Can you work these out from the model? Positions are in its coordinate system, mm. A direction names the side the tool comes from. Give positions to 0.01 mm unless a question says otherwise; leave off trailing zeros. Write each loop counter-clockwise with the first axis right and the second up, starting at its lowest first coordinate (ties: lowest second). Pieces come first, ordered by that corner, then holes. Notation, with made-up numbers: (9.5, 65.5) - (58.5, 65.5) arc R16 cw to (58.5, 88.5) - close; hole circle Ø8 at (-4, 33.5). An arc over 180 degrees is marked (long way). Use a Markdown table: item, result. Add a question column.
```python
from build123d import *

# Parameters (mm, degrees)
BOSS_EXTRUDE1_DEPTH = 128.5
SKETCH7_W           = 30
SKETCH7_H           = 20
BOSS_EXTRUDE4_DEPTH = 3
CUT_EXTRUDE1_REACH  = 145.152
SKETCH9_R           = 2.5
SKETCH10_W          = 20
SKETCH10_H          = 30
BOSS_EXTRUDE5_DEPTH = 3
CUT_EXTRUDE2_REACH  = 145.753
SKETCH11_R          = 2.5


with BuildPart() as part:
    # Sketch4 → Boss-Extrude1 (new, symmetric)
    with BuildSketch(Plane.XY):
        with BuildLine():
            Line((0, 0), (27, 0))
            Line((27, 0), (27, -3))
            Line((27, -3), (26.800082477, -3))
            ThreePointArc((26.800082477, -3), (-19.135504983, -19.08508544), (-3, 26.83281573))
            Line((-3, 26.83281573), (-3, 27))
            Line((-3, 27), (0, 27))
            Line((0, 27), (0, 0))
        make_face()
    extrude(amount=BOSS_EXTRUDE1_DEPTH, both=True)

    # Sketch7 → Boss-Extrude4 (add)
    with BuildSketch(Plane(origin=(0, 27, 0), x_dir=(1, 0, 0), z_dir=(0, 1, 0))):
        with Locations((12, -43.5)):
            Rectangle(SKETCH7_W, SKETCH7_H)
        with Locations((12, 43.5)):
            Rectangle(SKETCH7_W, SKETCH7_H)
    extrude(amount=BOSS_EXTRUDE4_DEPTH)

    # Sketch9 → Cut-Extrude1 (cut, up to next)
    with BuildSketch(Plane(origin=(0, 30, 0), x_dir=(1, 0, 0), z_dir=(0, 1, 0)), mode=Mode.PRIVATE) as cut_extrude1_sk1:
        with Locations(Location((17, -43.5, 0), (0, 0, 270))):
            Circle(SKETCH9_R)
    cut_extrude1_tool1 = extrude(cut_extrude1_sk1.sketch, amount=-CUT_EXTRUDE1_REACH, mode=Mode.PRIVATE) & part.part
    # Sketch9 → Cut-Extrude1 (cut, up to next)
    with BuildSketch(Plane(origin=(0, 30, 0), x_dir=(1, 0, 0), z_dir=(0, 1, 0)), mode=Mode.PRIVATE) as cut_extrude1_sk2:
        with Locations(Location((17, 43.5, 0), (0, 0, 270))):
            Circle(SKETCH9_R)
    cut_extrude1_tool2 = extrude(cut_extrude1_sk2.sketch, amount=-CUT_EXTRUDE1_REACH, mode=Mode.PRIVATE) & part.part
    add(cut_extrude1_tool1.solids().sort_by_distance((17, 30, 43.5))[0], mode=Mode.SUBTRACT)
    add(cut_extrude1_tool2.solids().sort_by_distance((17, 30, -43.5))[0], mode=Mode.SUBTRACT)

    # Sketch10 → Boss-Extrude5 (add)
    with BuildSketch(Plane(origin=(27, 0, 0), x_dir=(0, 0, -1), z_dir=(1, 0, 0))):
        with Locations((1.5, 12)):
            Rectangle(SKETCH10_W, SKETCH10_H)
    extrude(amount=BOSS_EXTRUDE5_DEPTH)

    # Sketch11 → Cut-Extrude2 (cut, up to next)
    with BuildSketch(Plane(origin=(30, 0, 0), x_dir=(0, 0, -1), z_dir=(1, 0, 0)), mode=Mode.PRIVATE) as cut_extrude2_sk1:
        with Locations((1.5, 17)):
            Circle(SKETCH11_R)
    cut_extrude2_tool1 = extrude(cut_extrude2_sk1.sketch, amount=-CUT_EXTRUDE2_REACH, mode=Mode.PRIVATE) & part.part
    add(cut_extrude2_tool1.solids().sort_by_distance((30, 17, -1.5))[0], mode=Mode.SUBTRACT)


solid = part.part
```
Q1. Suppose I cut it at A-A (z = -43.5). Please give me the cut outline in (x, y).
Q2. I'm going to push flat-ended pins straight in: P1, Ø1.5, axis at x = -1, z = -82, coming from the +Y side; P2, Ø0.9, axis at x = 28, y = 6, coming from the +Z side; P3, Ø5, axis at x = -21, z = -19, coming from the -Y side; P4, Ø6, axis at y = 17, z = -1.5, coming from the +X side. Where does each tip first touch, or does it pass through?
Q3. If we mould it in two halves opening along Y, with no side actions, what happens to faces 4 (the flat face through (12, 30, -44)), 5 (the cylindrical face through (-18.5, -19.7, 1.8)), 6 (the flat face through (13, 27, 43))? For each: released by +Y, released by -Y, zero draft, split by the parting line, or undercut.
Q4. Suppose I cut it at D-D (x = 9). Please give me the cut outline in (y, z).
Q5. On a 3-axis mill with a long thin cutter (end or side, diameter ignored), from which of +Z, -Z, +X, -X, +Y, -Y can I reach the whole of each face in a straight line? I mean faces 1 (the flat face through (27, 14, -1)), 2 (the flat face through (13, 27, -44)), 3 (the cylindrical face through (17.751, 28.521, 45.885)). Say none if no direction works.
Q6. If I drill on probe 1 along X at (y, z) = (27.7, 43.5); probe 2 along Y at (x, z) = (1, 36); probe 3 along X at (y, z) = (-1.5, -111.5), over which ranges is the centre line in solid material (lowest first)? Write a range as [from, to].
Q7. Suppose I cut it at C-C (z = 107). Please give me the cut outline in (x, y), and give its area (3 significant figures).
Q8. Suppose I cut it at B-B (y = 10.5). Please give me the cut outline in (x, z).
Derived:
| question | item | result |
|---|---|---|
| 1 | outline | (-3, 26.83) arc R27 ccw (long way) to (26.8, -3) - (27, -3) - (27, 0) - (0, 0) - (0, 27) - (14.5, 27) - (14.5, 30) - (-3, 30) - close; (19.5, 27) - (27, 27) - (27, 30) - (19.5, 30) - close |
| 2 | P1 | y = 27 |
| 2 | P2 | z = 8.5 |
| 2 | P3 | y = -19.7 |
| 2 | P4 | x = 30 |
| 3 | face 4 | released by +Y |
| 3 | face 5 | split by the parting line |
| 3 | face 6 | undercut |
| 4 | outline | (-25.45, -128.5) - (0, -128.5) - (0, 128.5) - (-25.45, 128.5) - close; (27, -53.5) - (30, -53.5) - (30, -33.5) - (27, -33.5) - close; (27, 33.5) - (30, 33.5) - (30, 53.5) - (27, 53.5) - close |
| 5 | face 1 | +Z, -Z, +Y |
| 5 | face 2 | +Z, -Z, +X |
| 5 | face 3 | +Y |
| 6 | probe 1 | [-3, 14.5], [19.5, 27] |
| 6 | probe 2 | [-26.98, 0], [27, 30] |
| 6 | probe 3 | [-26.99, 27] |
| 7 | outline | (-3, 26.83) arc R27 ccw (long way) to (26.8, -3) - (27, -3) - (27, 0) - (0, 0) - (0, 27) - (-3, 27) - close |
| 7 | area | 1,720 mm² |
| 8 | outline | (-24.91, -128.5) - (0, -128.5) - (0, 128.5) - (-24.91, 128.5) - close; (27, -11.5) - (30, -11.5) - (30, 8.5) - (27, 8.5) - close |
